Input: part model. Units: mm. Frame: model coordinates. A direction names the side the tool comes from. Coordinates: 2 decimals unless noted, no trailing zeros. Order: outer loops, then holes, each group sorted by start corner. A loop starts at its lowest first (then second) coordinate and runs counter-clockwise, first axis right, second up. Notation, with made-up numbers: M 32,89 L 83,89 A38 ccw 83,128 Z; hole C 81,71 d7. An arc over 180 degrees is marked long. Answer in a Markdown table with one row per item.
from build123d import *

# Parameters (mm, degrees)
SKETCH_2_R              = 1.5
EXTRUDE_1_DEPTH         = 10
FILLET_1_R              = 1.5
CUT_EXTRUDE_START       = 8.978636738
CUT_EXTRUDE_6_OUTLINE_W = 18
CUT_EXTRUDE_6_OUTLINE_H = 1
CUT_EXTRUDE_6_DEPTH     = 12.065744551
EXTRUDE_START           = -10
EXTRUDE_2_DEPTH         = 10


# Read off the part's stored shape, not the designer's step: 切除-拉伸6
with BuildPart() as part:
    # 草图2 → 凸台-拉伸1 (new body)
    with BuildSketch(Plane.XY):
        with BuildLine():
            Line((-3.738313135, -26.487804482), (8.522639585, -25.945713856))
            ThreePointArc((8.522639585, -25.945713856), (14.597644225, -30.744268797), (21.698305683, -33.828489568))
            Line((21.698305683, -33.828489568), (28.148131868, -29.931317342))
            ThreePointArc((28.148131868, -29.931317342), (11.679291726, -22.010339454), (5, -5))
            Line((5, -5), (5, 0))
            ThreePointArc((5, 0), (0, 5), (-5, 0))
            Line((-5, 0), (-5, -5))
            Line((-5, -5), (1.011e-06, -5))
            ThreePointArc((1.011e-06, -5), (0.486326168, -10.379869542), (1.929534162, -15.585314685))
            Line((1.929534162, -15.585314685), (-3.738313135, -26.487804482))
        make_face()
        Circle(SKETCH_2_R, mode=Mode.SUBTRACT)
    extrude(amount=EXTRUDE_1_DEPTH)

    # 圆角1
    fillet_1_edges = [part.edges().sort_by_distance(p)[0] for p in [
        (-3.738313135, -26.487804482, 5),
        (1.929534162, -15.585314685, 5),
        (-5, -5, 5),
        (28.148131868, -29.931317342, 5),
        (21.698305683, -33.828489568, 5),
        (8.522639585, -25.945713856, 5),
    ]]
    fillet(fillet_1_edges, radius=FILLET_1_R)

    # 切除-拉伸6 outline → 切除-拉伸6 (cut)
    with BuildSketch(Plane.YZ.offset(CUT_EXTRUDE_START)):
        with Locations((-26, 5)):
            Rectangle(CUT_EXTRUDE_6_OUTLINE_W, CUT_EXTRUDE_6_OUTLINE_H)
    extrude(amount=CUT_EXTRUDE_6_DEPTH, mode=Mode.SUBTRACT)

    # 草图3 → 凸台-拉伸2 (add)
    with BuildSketch(Plane.XY.offset(10).offset(EXTRUDE_START)):
        with BuildLine():
            Line((-2.473670042, -25.681158433), (-1.937795126, -25.681158433))
            ThreePointArc((-1.937795126, -25.681158433), (-3.071581107, -18.689223974), (1.070755407, -12.943471949))
            ThreePointArc((1.070755407, -12.943471949), (0.992362696, -12.652249172), (0.916901566, -12.360253041))
            ThreePointArc((0.916901566, -12.360253041), (-3.537234076, -18.318495365), (-2.473670042, -25.681158433))
        make_face()
    extrude(amount=EXTRUDE_2_DEPTH)


solid = part.part
1) Cut plane C-C, the plane x = -2. Output: boundary loops of the cut face in (y, z).
Resolved:
| item | result |
|---|---|
| outline | M -26.15,0 L -23.14,0 L -23.14,10 L -26.15,10 Z; M -16.05,0 L -15.03,0 L -15.03,10 L -16.05,10 Z; M -5,0 L 4.58,0 L 4.58,10 L -5,10 Z |
2) Cut plane A-A, the plane z = 5. Output: boundary loops of the cut face in (x, y), and give its area (3 significant figures).
Resolved:
| item | result |
|---|---|
| outline | M -5,-3.5 A1.5 ccw -3.5,-5 L 0,-5 A30 ccw 0.92,-12.36 A9.72 ccw -2.53,-25.58 A1.5 ccw -1.14,-26.37 L 7.86,-25.97 A1.5 cw 8.98,-26.4 L 8.98,-18.53 A25 cw 5,-5 L 5,0 A5 ccw -5,0 Z; M 21.04,-33.63 A1.5 ccw 22.27,-33.48 L 24.62,-32.06 A1.5 ccw 24.2,-29.32 A25 cw 21.04,-28.34 Z; hole M -2.62,-24.36 A1.5 cw -2.54,-24.18 L 1.63,-16.17 A1.5 ccw 1.71,-14.98 A30 cw 1.07,-12.94 A9.25 ccw Z; hole C 0,0 d3 |
| area | 260 mm2 |
3) Mould query, pull axis Y, two halves, no side actions, for faces 1 (the face through (-2.9, -18.06, 4.93)), 2 (the face through (15, -26, 5.5)), 3 (the face through (1.79, -15.59, 5.07)), 4 (the face through (21.66, -33.69, 5.07)). Classes: +Y half, -Y half, draft (parallel to the pull), parting line (faces both ways), or undercut.
Resolved:
| item | result |
|---|---|
| face 1 | undercut |
| face 2 | draft |
| face 3 | undercut |
| face 4 | -Y half |
4) Cut plane D-D, the plane z = 8. Output: boundary loops of the cut face in (x, y), and give its area (3 significant figures).
Resolved:
| item | result |
|---|---|
| outline | M -5,-3.5 A1.5 ccw -3.5,-5 L 0,-5 A30 ccw 0.92,-12.36 A9.72 ccw -2.53,-25.58 A1.5 ccw -1.14,-26.37 L 7.86,-25.97 A1.5 cw 8.98,-26.4 A30 ccw 21.04,-33.63 A1.5 ccw 22.27,-33.48 L 24.62,-32.06 A1.5 ccw 24.2,-29.32 A25 cw 5,-5 L 5,0 A5 ccw -5,0 Z; hole M -2.62,-24.36 A1.5 cw -2.54,-24.18 L 1.63,-16.17 A1.5 ccw 1.71,-14.98 A30 cw 1.07,-12.94 A9.25 ccw Z; hole C 0,0 d3 |
| area | 334 mm2 |
5) Reachability of faces 5 (the face through (15, -26, 4.5)), 6 (the face through (3.296, -26.177, 4.93)), 7 (the face through (5, -3, 5)) from +Z, -Z, +X, -X, +Y, -Y: full face, straight path, thin tool, end or side. Return the list, or none.
Resolved:
| item | result |
|---|---|
| face 5 | +Y, -Y |
| face 6 | +Z, -Z, -Y |
| face 7 | +Z, -Z, +X, +Y |
6) Contact query for flat-ended pins moving along their axis: pin 1 (2 mm diameter, centred on y = -20.5, z = 6.5, fed in from +X); pin 2 (6 mm diameter, centred on y = -11, z = 4, fed in from +X); pin 3 (1.1 mm diameter, centred on x = -2.5, z = 7, fed in from -Y); pin 4 (1.8 mm diameter, centred on x = 0, y = 0, fed in from -Z). Output: stop coordinate, or through.
Resolved:
| item | result |
|---|---|
| pin 1 | stops at x = 11.22 |
| pin 2 | stops at x = 6.68 |
| pin 3 | stops at y = -26.18 |
| pin 4 | passes through |
7) Cut plane B-B, the plane y = -21.5. Output: boundary loops of the cut face in (x, z).
Resolved:
| item | result |
|---|---|
| outline | M -3.81,0 L -3.29,0 L -3.29,10 L -3.81,10 Z; M -1.15,0 L 11.22,0 L 11.22,4.5 L 8.98,4.5 L 8.98,5.5 L 11.22,5.5 L 11.22,10 L -1.15,10 Z |
8) Material intervals for probe 1 along Z at (x, y) = (11, -28); probe 2 along Y at (x, z) = (1, 1); probe 3 along X at (y, z) = (-15, 6.75), sorted ascending.
Resolved:
| item | result |
|---|---|
| probe 1 | z = 0 to 4.5, 5.5 to 10 |
| probe 2 | y = -26.28 to -17.37, -12.99 to -1.12, 1.12 to 4.9 |
| probe 3 | x = -1.98 to -1.26, 1.72 to 7.09 |
